Design review of the part built by this model. Coordinates are the model's own, in mm. Face numbers are marked on the shaded views. A direction names the side the tool comes from. Coordinates: 2 decimals unless noted, no trailing zeros. Write each loop counter-clockwise with the first axis right and the second up, starting at its lowest first coordinate (ties: lowest second). Pieces come first, ordered by that corner, then holes.
Q1. Add section B-B, the plane y = 20. Give the boundary of the cut face in (x, z).
Q2. Machinability: for the marked faces 4 and 5, which of the approach directions +Z, -Z, +X, -X, +Y, -Y give a long, thin tool a straight path to every point of the face, cutting with its end or side? Answer none if there is none.
Q3. Add section A-A, the plane z = 7.25. Give the boundary of the cut face in (x, y), plus the area to 3 significant figures.
Q4. The part is to be moulded in two halves that separate along X. For the marked faces 1, 2 and 3, say which applies: +X half, -X half, draft (parallel to the pull), parting line (faces both ways), or undercut.
Q5. Add section C-C, the plane x = 11. Give the boundary of the cut face in (y, z).
Q6. Add section D-D, the plane y = 11.5. Give the boundary of the cut face in (x, z).
Q7. To check wall thickness, follow probe 1 along X at (y, z) = (23.5, 15.25); probe 2 along Y at (x, z) = (36, 5); probe 3 along X at (y, z) = (19, 3). State the ranges of each line that lie inside material, in increasing order.
Q8. Clearance check with flat-ended pins moving along their axes: pin 1 Ø1 at (y, z) = (17, 9) entering from -X; pin 2 Ø6 at (y, z) = (2.5, 15) entering from -X; pin 3 Ø10 at (x, z) = (16.5, 14) entering from +Y; pin 4 Ø5.5 at (x, y) = (36.6, 21.56) entering from +Z. State where each tip first meets the part, or that it passes through.
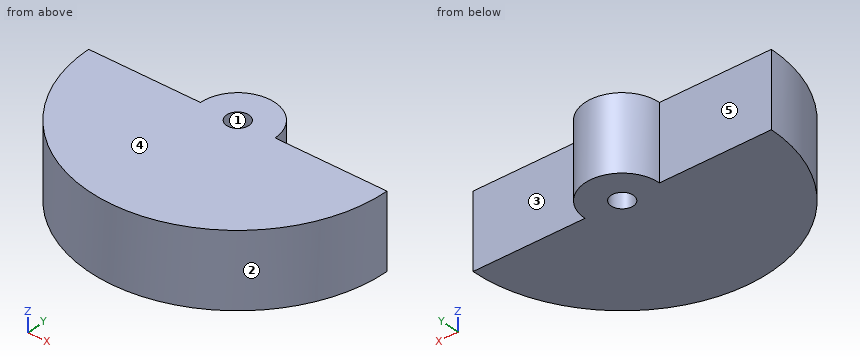
from build123d import *

# Parameters (mm, degrees)
BOSS_EXTRUDE1_DEPTH = 20
SKETCH2_R           = 10
BOSS_EXTRUDE2_DEPTH = 20
SKETCH3_R           = 3
CUT_EXTRUDE1_DEPTH  = 20


with BuildPart() as part:
    # Sketch1 → Boss-Extrude1 (new body)
    with BuildSketch(Plane.XY):
        with BuildLine():
            Line((-3.402685511, 21.555471253), (76.597314489, 21.555471253))
            ThreePointArc((76.597314489, 21.555471253), (36.597314489, -18.444528747), (-3.402685511, 21.555471253))
        make_face()
    extrude(amount=BOSS_EXTRUDE1_DEPTH)

    # Sketch2 → Boss-Extrude2 (add)
    with BuildSketch(Plane(origin=(0, 0, 0), x_dir=(-1, 0, 0), z_dir=(0, 0, -1))):
        with Locations((-36.597314489, 21.555471253)):
            Circle(SKETCH2_R)
    extrude(amount=-BOSS_EXTRUDE2_DEPTH)

    # Sketch3 → Cut-Extrude1 (cut)
    with BuildSketch(Plane(origin=(0, 0, 0), x_dir=(-1, 0, 0), z_dir=(0, 0, -1))):
        with Locations((-36.597314489, 21.555471253)):
            Circle(SKETCH3_R)
    extrude(amount=-CUT_EXTRUDE1_DEPTH, mode=Mode.SUBTRACT)


solid = part.part
Here are the results:
1. outline: (-3.37, 0) - (34.03, 0) - (34.03, 20) - (-3.37, 20) - close; (39.16, 0) - (76.57, 0) - (76.57, 20) - (39.16, 20) - close
2. face 4: +Z, +X, -X, +Y, -Y
2. face 5: +Z, -Z, -X, +Y
3. outline: (-3.4, 21.56) arc R40 ccw to (76.6, 21.56) - (46.6, 21.56) arc R10 ccw to (26.6, 21.56) - close; hole circle Ø6 at (36.6, 21.56)
3. area: 2,640 mm2
4. face 1: undercut
4. face 2: parting line
4. face 3: draft
5. outline: (-9.18, 0) - (21.56, 0) - (21.56, 20) - (-9.18, 20) - close
6. outline: (-2.12, 0) - (75.31, 0) - (75.31, 20) - (-2.12, 20) - close
7. probe 1: x = 26.79 to 34.31, 38.88 to 46.41
7. probe 2: y = -18.44 to 18.62, 24.5 to 31.54
7. probe 3: x = -3.32 to 35.03, 38.17 to 76.52
8. pin 1: stops at x = -3.2
8. pin 2: stops at x = -0.04
8. pin 3: stops at y = 21.56
8. pin 4: passes through
